For this review, take the finished solid that the model builds, in its own axes (mm). Give positions to 0.01 mm unless a question says otherwise; leave off trailing zeros. Write each loop counter-clockwise with the first axis right and the second up, starting at its lowest first coordinate (ties: lowest second). Pieces come first, ordered by that corner, then holes. Notation, with made-up numbers: M 6.5,29.25 L 17.5,29.25 A29 cw 17.5,55.25 Z; hole C -34,-29.75 d8. An arc over 180 degrees is marked long. Answer as a JSON object with one key per item and string values. Group by question number.
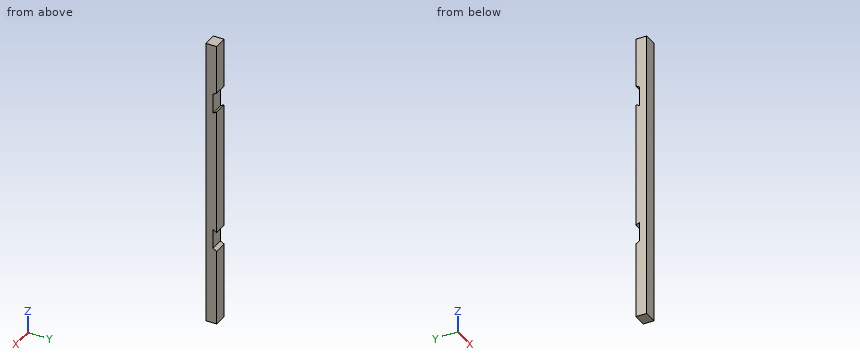
```python
from build123d import *

# Parameters (mm, degrees)
F2_DEPTH = 50


# Not quite as in the source:
# - a feature names something its author has since deleted; it is built from what else it names


with BuildPart() as f2:
    # F1 (on Right) → F2 (new body)
    with BuildSketch(Plane.YZ):
        Polygon((-26.6666666667, 40), (-26.6666666667, 220), (-66.6666666667, 220), (-66.6666666667, -850), (-26.6666666667, -850), (-26.6666666667, -570), (-40, -562.3019964108), (-40, -490), (-26.6666666667, -497.6980035892), (-26.6666666667, -32.3019964108), (-40, -40), (-40, 32.3019964108), align=None)
    extrude(amount=F2_DEPTH)


solid = f2.part
```
Item 1: Consider section A-A (x = 41.5). Give the boundary of the cut face in (y, z).
Item 2: To check wall thickness, follow probe 1 along Z at (x, y) = (12.5, -34.5); probe 2 along Z at (x, y) = (46, -28.5); probe 3 along Y at (x, z) = (5, -557). State the ranges of each line that lie inside material, in increasing order.
Item 3: Insertion check: P1, Ø25, axis at x = 34.5, z = -16, coming from the +Y side. The pin has a flat end and moves straight along its axis. Give the tip position at first contact, or say it passes through.
Result set:
{
 "1": {"outline": "M -66.67,-850 L -26.67,-850 L -26.67,-570 L -40,-562.3 L -40,-490 L -26.67,-497.7 L -26.67,-32.3 L -40,-40 L -40,32.3 L -26.67,40 L -26.67,220 L -66.67,220 Z"},
 "2": {"probe 1": "z = -850 to -565.48, -493.18 to -36.82, 35.48 to 220", "probe 2": "z = -850 to -568.94, -496.64 to -33.36, 38.94 to 220", "probe 3": "y = -66.67 to -40"},
 "3": {"P1": "stops at y = -40"}
}
